from build123d import *

# Parameters (mm, degrees)
ESQUISSE1_R             = 9
ESQUISSE1_R_2           = 1.1
ESQUISSE1_R_3           = 4
BOSS_EXTRU_1_DEPTH      = 2
BOSS_EXTRU_2_START      = -2
ESQUISSE2_R             = 3
BOSS_EXTRU_2_DEPTH      = 2
ENL_V_MAT_EXTRU_1_DEPTH = 47.52268264
CONG_1_R                = 2
ESQUISSE4_R             = 1.5
BOSS_EXTRU_3_DEPTH      = 2


with BuildPart() as part:
    # Esquisse1 → Boss.-Extru.1 (new body)
    with BuildSketch(Plane.XY):
        Circle(ESQUISSE1_R)
        with Locations((0, 6)):
            Circle(ESQUISSE1_R_2, mode=Mode.SUBTRACT)
        with Locations((6, 0)):
            Circle(ESQUISSE1_R_2, mode=Mode.SUBTRACT)
        with Locations((0, -6)):
            Circle(ESQUISSE1_R_2, mode=Mode.SUBTRACT)
        with Locations((-6, 0)):
            Circle(ESQUISSE1_R_2, mode=Mode.SUBTRACT)
        Circle(ESQUISSE1_R_3, mode=Mode.SUBTRACT)
    extrude(amount=BOSS_EXTRU_1_DEPTH)

    # Esquisse2 → Boss.-Extru.2 (add)
    with BuildSketch(Plane.XY.offset(2).offset(BOSS_EXTRU_2_START)):
        with BuildLine():
            Line((0.765, 8.967428561), (40.476, 5.579733327))
            ThreePointArc((40.476, 5.579733327), (45.6, 0), (40.476, -5.579733327))
            Line((40.476, -5.579733327), (0.765, -8.967428561))
            ThreePointArc((0.765, -8.967428561), (9, 0), (0.765, 8.967428561))
        make_face()
        with Locations((40, 0)):
            Circle(ESQUISSE2_R, mode=Mode.SUBTRACT)
    extrude(amount=BOSS_EXTRU_2_DEPTH)

    # Esquisse3 → Enlèv. mat.-Extru.1 (cut, through all)
    with BuildSketch(Plane.XY.offset(2)):
        with BuildLine():
            Line((7.193926615, 5.408088373), (35.279111191, 3.012176763))
            ThreePointArc((35.279111191, 3.012176763), (34.4, 0), (35.279111191, -3.012176763))
            Line((35.279111191, -3.012176763), (7.193926615, -5.408088373))
            ThreePointArc((7.193926615, -5.408088373), (9, 0), (7.193926615, 5.408088373))
        make_face()
    extrude(amount=-ENL_V_MAT_EXTRU_1_DEPTH, mode=Mode.SUBTRACT)

    # Congé1
    cong_1_edges = [part.edges().sort_by_distance(p)[0] for p in [
        (7.193926615, -5.408088373, 1),
        (7.193926615, 5.408088373, 1),
        (35.279111191, 3.012176763, 1),
        (35.279111191, -3.012176763, 1),
    ]]
    fillet(cong_1_edges, radius=CONG_1_R)

    # Esquisse4 → Boss.-Extru.3 (add)
    with BuildSketch(Plane.XY.offset(2)):
        with BuildLine():
            Line((42.146666667, 5.172216374), (52.383333333, 0.923610067))
            ThreePointArc((52.383333333, 0.923610067), (53, 0), (52.383333333, -0.923610067))
            Line((52.383333333, -0.923610067), (42.146666667, -5.172216374))
            ThreePointArc((42.146666667, -5.172216374), (45.6, 0), (42.146666667, 5.172216374))
        make_face()
        with Locations((48, 0)):
            Circle(ESQUISSE4_R, mode=Mode.SUBTRACT)
    extrude(amount=-BOSS_EXTRU_3_DEPTH)


solid = part.part
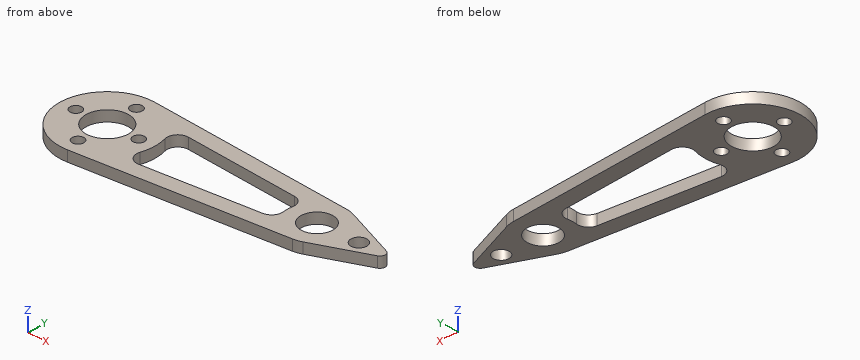
CAD build for the part. Positions are in the model's coordinates, mm. Coordinates: 2 decimals unless noted, no trailing zeros. Loops run counter-clockwise (first coordinate to the right, second up) from the corner with the lowest first, then second, coordinate; pieces in that order, holes last. Notation, with made-up numbers: (42, -38) - (90, -38) arc R13 ccw to (90, -17) - close; hole circle Ø4 at (84, -4.75). An arc over 180 degrees is marked (long way). Use one line per item in the form item = value. Start each with the question number.
1) Drill centre lines: L1, parallel to Y at x = 0, z = 1.6; L2, parallel to X at y = 1.75, z = 1.35; L3, parallel to Y at x = 6, z = 1.45. Where is each one in solid material? Low to high. Write a range as from..to.
2) Band-saw the part on A-A (y = 0). Give the cut face in (x, z), and give its area (3 significant figures).
3) Band-saw the part on B-B (x = 0). Give the cut face in (y, z), and give its area (3 significant figures).
4) Band-saw the part on C-C (z = 1.7). State how many separate pieces and enclosed holes the cut face has, and give its area (3 significant figures).
5) Band-saw the part on D-D (x = 18.5). Give the cut face in (y, z).
Check values:
q1.L1 = -9..-7.1, -4.9..-4, 4..4.9, 7.1..9
q1.L2 = -8.83..-3.6, 3.6..8.83, 34.44..37.56, 42.44..50.39
q1.L3 = -8.52..-1.1, 1.1..8.52
q2.outline = (-9, 0) - (-7.1, 0) - (-7.1, 2) - (-9, 2) - close; (-4.9, 0) - (-4, 0) - (-4, 2) - (-4.9, 2) - close; (4, 0) - (4.9, 0) - (4.9, 2) - (4, 2) - close; (7.1, 0) - (9, 0) - (9, 2) - (7.1, 2) - close; (34.4, 0) - (37, 0) - (37, 2) - (34.4, 2) - close; (43, 0) - (46.5, 0) - (46.5, 2) - (43, 2) - close; (49.5, 0) - (53, 0) - (53, 2) - (49.5, 2) - close
q2.area = 30.4 mm2
q3.outline = (-9, 0) - (-7.1, 0) - (-7.1, 2) - (-9, 2) - close; (-4.9, 0) - (-4, 0) - (-4, 2) - (-4.9, 2) - close; (4, 0) - (4.9, 0) - (4.9, 2) - (4, 2) - close; (7.1, 0) - (9, 0) - (9, 2) - (7.1, 2) - close
q3.area = 11.2 mm2
q4.separate_pieces = 1
q4.enclosed_holes = 8
q4.area = 487 mm2
q5.outline = (-7.45, 0) - (-4.44, 0) - (-4.44, 2) - (-7.45, 2) - close; (4.44, 0) - (7.45, 0) - (7.45, 2) - (4.44, 2) - close
